from build123d import *

# Parameters (mm, degrees)
F1_DEPTH       = 7.5
F3_D           = 3
F3_CBORE_D     = 6
F3_CBORE_DEPTH = 2.2
F5_DEPTH       = 3
F9_DEPTH       = 18.501
F9_DEPTH_BACK  = 16.501


with BuildPart() as f1:
    # F0 (on Top) → F1 (new body, symmetric)
    with BuildSketch(Plane.XY):
        with BuildLine():
            Line((-16, 18.5), (-16, 12.5))
            Line((-16, 12.5), (-1.5, 12.5))
            ThreePointArc((-1.5, 12.5), (-0.4393398282, 12.0606601718), (0, 11))
            Line((0, 11), (0, -9))
            ThreePointArc((0, -9), (-0.4393398282, -10.0606601718), (-1.5, -10.5))
            Line((-1.5, -10.5), (-16, -10.5))
            Line((-16, -10.5), (-16, -16.5))
            Line((-16, -16.5), (10, -16.5))
            Line((10, -16.5), (10, 3.5))
            Line((10, 3.5), (7, 3.5))
            Line((7, 3.5), (7, -4))
            Line((7, -4), (6, -4))
            Line((6, -4), (6, 18.5))
            Line((6, 18.5), (-16, 18.5))
        make_face()
    extrude(amount=F1_DEPTH, both=True)

    # F3 (through all)
    with Locations(Plane(origin=(0, 0, 0), x_dir=(0, -1, 0), z_dir=(-1, 0, 0))):
        with Locations((0, 0)):
            CounterBoreHole(F3_D / 2, F3_CBORE_D / 2, F3_CBORE_DEPTH)

    # F4 (on face) → F5 (cut, through all)
    with BuildSketch(Plane.YZ.offset(10)):
        with BuildLine():
            Line((2, 3), (0, 3))
            ThreePointArc((0, 3), (-3, 0), (0, -3))
            Line((0, -3), (2, -3))
            Line((2, -3), (2, 3))
        make_face()
    extrude(amount=-F5_DEPTH, mode=Mode.SUBTRACT)

    # F6 (on Top) → F7 (revolve, cut)
    with BuildSketch(Plane.XY):
        Polygon((-9, -16.5), (-4, -16.5), (-4, -13.9), (-6.25, -13.9), (-6.25, 15.9), (-4, 15.9), (-4, 18.5), (-9, 18.5), align=None)
    revolve(axis=Axis((-9, 21, 0), (0, 1, 0)), mode=Mode.SUBTRACT)

    # F8 (on Front) → F9 (cut, two sides)
    with BuildSketch(Plane.XZ) as f9_sk:
        with BuildLine():
            ThreePointArc((-14.5404962177, -7.5), (-16, 0), (-14.5404962177, 7.5))
            Line((-14.5404962177, 7.5), (-17.27, 7.5))
            Line((-17.27, 7.5), (-17.27, -7.5))
            Line((-17.27, -7.5), (-14.5404962177, -7.5))
        make_face()
    extrude(amount=-F9_DEPTH, mode=Mode.SUBTRACT)
    extrude(f9_sk.sketch, amount=F9_DEPTH_BACK, mode=Mode.SUBTRACT)


solid = f1.part
Geometry check sheet. Reference: the model listing, model coordinates, mm. A direction names the side the tool comes from. Round coordinates to 2 decimals unless told otherwise and drop trailing zeros. Order: outer loops, then holes, each group sorted by start corner. A loop starts at its lowest first (then second) coordinate and runs counter-clockwise, first axis right, second up. Notation, with made-up numbers: M 44,39.25 L 95,39.25 A20 ccw 95,61.25 Z; hole C 51,45 d8. An arc over 180 degrees is marked long. Answer in a Markdown table with one row per item. Add a question column.
Item 1: Draft check along Y on faces 1 (the face through (1, 3, 0)), 2 (the face through (-6.8, -13.9, 2.2)), 3 (the face through (-2, 18.5, 0)). Enter one of: released by +Y, released by -Y, zero draft, split by the parting line, or undercut.
Item 2: Depth check by flat-ended pin: pin 1 Ø3 at (x, z) = (-11, 2.5) entering from +Y; pin 2 Ø2.5 at (x, z) = (8.5, -0.5) entering from +Y; pin 3 Ø4 at (y, z) = (-0.5, -3.5) entering from -X. Enter the tip coordinate at first touch or a pass-through.
Item 3: Material ranges on L1, parallel to Z at x = -9, y = 16.55; L2, parallel to Z at x = -9, y = 13.4; L3, parallel to X at y = 1.5, z = 6.5, recorded low to high. Write a range as [from, to].
Item 4: Sectioned sample at D-D, the plane x = -3.5. Enter the section's corners in (y, z).
Item 5: Sectioned sample at C-C, the plane y = -1. Enter the section's corners in (x, z), plus the area to 3 significant figures.
Item 6: Set-up check for faces 4 (the face through (9, 1, -3)), 5 (the face through (2.2, -1.3, -1.3)), 6 (the face through (-11.2, 15.9, 2.2)), 7 (the face through (-5, -10.5, 0)), 8 (the face through (7, 2.3, 0.1)): record each of +Z, -Z, +X, -X, +Y, -Y from which the full face is reachable in a straight line by a thin tool's end or side.
Item 7: Sectioned sample at A-A, the plane x = -9. Enter the section's corners in (y, z), plus the area to 3 significant figures.
Item 8: Sectioned sample at B-B, the plane x = 7.5. Enter the section's corners in (y, z), plus the area to 3 significant figures.
Filled in:
| question | item | result |
|---|---|---|
| 1 | face 1 | undercut |
| 1 | face 2 | released by -Y |
| 1 | face 3 | released by +Y |
| 2 | pin 1 | stops at y = 15.9 |
| 2 | pin 2 | stops at y = 3.5 |
| 2 | pin 3 | stops at x = 0 |
| 3 | L1 | z = [-7.5, -5], [5, 7.5] |
| 3 | L2 | z = [-7.5, -2.75], [2.75, 7.5] |
| 3 | L3 | x = [0, 6], [7, 10] |
| 4 | outline | M -16.5,-7.5 L -10.5,-7.5 L -10.5,7.5 L -16.5,7.5 Z; M 12.5,-7.5 L 18.5,-7.5 L 18.5,7.5 L 12.5,7.5 Z |
| 5 | outline | M 0,-7.5 L 6,-7.5 L 6,-1.12 L 2.2,-1.12 L 2.2,-2.83 L 0,-2.83 Z; M 0,2.83 L 2.2,2.83 L 2.2,1.12 L 6,1.12 L 6,7.5 L 0,7.5 Z; M 7,-7.5 L 10,-7.5 L 10,-2.83 L 7,-2.83 Z; M 7,2.83 L 10,2.83 L 10,7.5 L 7,7.5 Z |
| 5 | area | 97.1 mm² |
| 6 | face 4 | +X |
| 6 | face 5 | -X |
| 6 | face 6 | +Y |
| 6 | face 7 | +Z, -Z, -X |
| 6 | face 8 | +Z, -Z, +Y |
| 7 | outline | M -16.5,-7.5 L -10.5,-7.5 L -10.5,-2.75 L -13.9,-2.75 L -13.9,-5 L -16.5,-5 Z; M -16.5,5 L -13.9,5 L -13.9,2.75 L -10.5,2.75 L -10.5,7.5 L -16.5,7.5 Z; M 12.5,-7.5 L 18.5,-7.5 L 18.5,-5 L 15.9,-5 L 15.9,-2.75 L 12.5,-2.75 Z; M 12.5,2.75 L 15.9,2.75 L 15.9,5 L 18.5,5 L 18.5,7.5 L 12.5,7.5 Z |
| 7 | area | 90.6 mm² |
| 8 | outline | M -16.5,-7.5 L 3.5,-7.5 L 3.5,7.5 L -16.5,7.5 Z; hole M 0,-3 L 2,-3 L 2,3 L 0,3 A3 ccw Z |
| 8 | area | 274 mm² |
